Here's how the part is built. I have some questions about the finished solid (model axes, mm). Face numbers are marked on the shaded views. A direction names the side the tool comes from. Coordinates: 2 decimals unless noted, no trailing zeros. Write each loop counter-clockwise with the first axis right and the second up, starting at its lowest first coordinate (ties: lowest second). Pieces come first, ordered by that corner, then holes. Notation, with made-up numbers: (27, -18.5) -> (67, -18.5) arc R32 cw to (67, 11.5) -> close; hole circle Ø7 at (57, -23.5). An arc over 180 degrees is marked (long way). Use a Markdown table: item, result. Add a question column.
Item 1: If we mould it in two halves opening along X, with no side actions, what happens to the marked faces 6, 7, 8 and 9? For each: pulls with the +X half, pulls with the -X half, needs draft (parallel to the pull), parting line crosses it, or undercut.
Item 2: Imagine slicing it at C-C, the plane z = 281.5. Write out the boundary of the cut face in (x, y).
Item 3: Imagine slicing it at A-A, the plane z = 61.5. Write out the boundary of the cut face in (x, y).
Item 4: On a 3-axis mill with a long thin cutter (end or side, diameter ignored), from which of +Z, -Z, +X, -X, +Y, -Y can I reach the whole of each face in a straight line? I mean the marked faces 1, 2, 3, 4 and 5. Say none if no direction works.
Item 5: Imagine slicing it at D-D, the plane y = 276. Write out the boundary of the cut face in (x, z), and give its area (3 significant figures).
Item 6: Will these pins go through, and if not, where does the flat tip stop? pin 1 Ø12 at (x, y) = (138.5, 3) entering from -Z; pin 2 Ø3 at (x, z) = (-128.5, -9) entering from -Y; pin 3 Ø8 at (y, z) = (170, -138) entering from +X.
Item 7: Imagine slicing it at B-B, the plane x = 521.5. Write out the boundary of the cut face in (y, z).
Item 8: If I drill on line 1 along Z through (x, y) = (-482.5, -20.5); line 2 along Z through (x, y) = (-534, -6); line 3 along Z through (x, y) = (-270, 265), over which ranges is the centre line in solid material (lowest first)? Write a range as from..to.
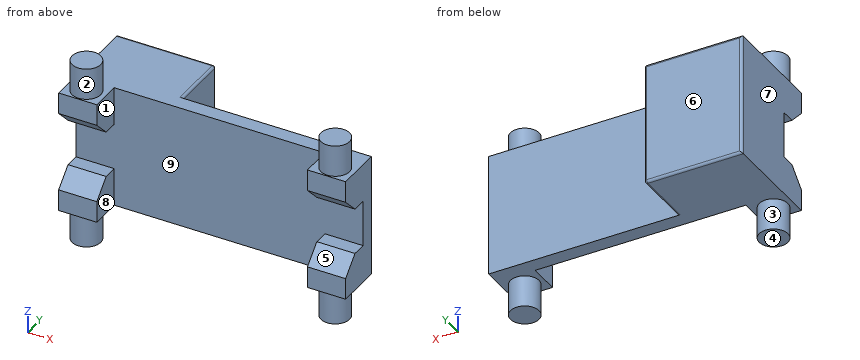
```python
from build123d import *

# Parameters (mm, degrees)
SKETCH_1_W      = 1203
SKETCH_1_H      = 514
EXTRUDE_1_DEPTH = 62
SKETCH_2_W      = 410
SKETCH_2_H      = 514
EXTRUDE_2_DEPTH = 250
FILLET_1_R      = 10
SKETCH_3_W      = 160
SKETCH_3_H      = 160
EXTRUDE_3_DEPTH = 130
CHAMFER_1_SIZE  = 70
SKETCH_5_R      = 60
EXTRUDE_4_DEPTH = 132
SKETCH_4_R      = 60
EXTRUDE_5_DEPTH = 132


with BuildPart() as part:
    # Эскиз1 → Бобышка-Вытянуть1 (new body)
    with BuildSketch(Plane(origin=(0, 0, 0), x_dir=(1, 0, 0), z_dir=(0, 1, 0))):
        Rectangle(SKETCH_1_W, SKETCH_1_H)
    extrude(amount=EXTRUDE_1_DEPTH)

    # Эскиз2 → Бобышка-Вытянуть2 (add)
    with BuildSketch(Plane(origin=(0, 62, 0), x_dir=(1, 0, 0), z_dir=(0, 1, 0))):
        with Locations((-396.5, 0)):
            Rectangle(SKETCH_2_W, SKETCH_2_H)
    extrude(amount=EXTRUDE_2_DEPTH)

    # Скругление1
    fillet_1_edges = [part.edges().sort_by_distance(p)[0] for p in [
        (-191.5, 187, 257),
        (-191.5, 187, -257),
        (-601.5, 312, 0),
        (-396.5, 312, 257),
        (-191.5, 312, 0),
        (-396.5, 312, -257),
    ]]
    fillet(fillet_1_edges, radius=FILLET_1_R)

    # Эскиз3 → Бобышка-Вытянуть3 (add)
    with BuildSketch(Plane.XZ):
        with Locations((-521.5, 177)):
            Rectangle(SKETCH_3_W, SKETCH_3_H)
        with Locations((-521.5, -177)):
            Rectangle(SKETCH_3_W, SKETCH_3_H)
        with Locations((521.5, -177)):
            Rectangle(SKETCH_3_W, SKETCH_3_H)
        with Locations((521.5, 177)):
            Rectangle(SKETCH_3_W, SKETCH_3_H)
    extrude(amount=EXTRUDE_3_DEPTH)

    # Фаска1
    chamfer_1_edges = [part.edges().sort_by_distance(p)[0] for p in [
        (521.5, -130, 97),
        (-521.5, -130, 97),
        (-521.5, -130, -97),
        (521.5, -130, -97),
    ]]
    chamfer(chamfer_1_edges, length=CHAMFER_1_SIZE)

    # Эскиз5 → Бобышка-Вытянуть4 (add)
    with BuildSketch(Plane(origin=(0, 0, -257), x_dir=(-1, 0, 0), z_dir=(0, 0, -1))):
        with Locations((521.5, -65)):
            Circle(SKETCH_5_R)
        with Locations((-521.5, -65)):
            Circle(SKETCH_5_R)
    extrude(amount=EXTRUDE_4_DEPTH)

    # Эскиз4 → Бобышка-Вытянуть5 (add)
    with BuildSketch(Plane.XY.offset(257)):
        with Locations((-521.5, -65)):
            Circle(SKETCH_4_R)
        with Locations((521.5, -65)):
            Circle(SKETCH_4_R)
    extrude(amount=EXTRUDE_5_DEPTH)


solid = part.part
```
Ans:
| question | item | result |
|---|---|---|
| 1 | face 6 | needs draft |
| 1 | face 7 | pulls with the -X half |
| 1 | face 8 | undercut |
| 1 | face 9 | undercut |
| 2 | outline | circle Ø120 at (-521.5, -65); circle Ø120 at (521.5, -65) |
| 3 | outline | (-601.5, 0) -> (601.5, 0) -> (601.5, 62) -> (-191.5, 62) -> (-191.5, 302) arc R10 ccw to (-201.5, 312) -> (-591.5, 312) arc R10 ccw to (-601.5, 302) -> close |
| 4 | face 1 | +Z, -Z, -Y |
| 4 | face 2 | +Z |
| 4 | face 3 | -Z |
| 4 | face 4 | -Z, +X, -X, +Y, -Y |
| 4 | face 5 | +X, -X, -Y |
| 5 | outline | (-601.5, -257) -> (-201.5, -257) arc R10 ccw to (-191.5, -247) -> (-191.5, 247) arc R10 ccw to (-201.5, 257) -> (-601.5, 257) -> close |
| 5 | area | 211,000 mm^2 |
| 6 | pin 1 | stops at z = -257 |
| 6 | pin 2 | stops at y = 0 |
| 6 | pin 3 | stops at x = -191.5 |
| 7 | outline | (-130, -257) -> (-125, -257) -> (-125, -389) -> (-5, -389) -> (-5, -257) -> (62, -257) -> (62, 257) -> (-5, 257) -> (-5, 389) -> (-125, 389) -> (-125, 257) -> (-130, 257) -> (-130, 167) -> (-60, 97) -> (0, 97) -> (0, -97) -> (-60, -97) -> (-130, -167) -> close |
| 8 | line 1 | z = -389..-97, 97..389 |
| 8 | line 2 | z = -257..-97, 97..257 |
| 8 | line 3 | z = -257..257 |
